from build123d import *

# Parameters (mm, degrees)
SKETCH1_W           = 42
SKETCH1_H           = 16
BOSS_EXTRUDE1_DEPTH = 7
SKETCH2_R           = 1
BOSS_EXTRUDE2_DEPTH = 1.6
CUT_EXTRUDE1_REACH  = 26.062
SKETCH3_R           = 1.45
BOSS_EXTRUDE3_DEPTH = 16
CUT_EXTRUDE2_REACH  = 72.718
SKETCH5_R           = 2.75
BOSS_EXTRUDE4_DEPTH = 6
CUT_EXTRUDE3_DEPTH  = 8
FILLET1_R           = 5
CHAMFER2_SIZE       = 3
CHAMFER3_SIZE       = 15
CHAMFER5_SIZE       = 20
SKETCH8_W           = 16
SKETCH8_H           = 4
SKETCH8_W_2         = 6
SKETCH8_H_2         = 10
CUT_EXTRUDE4_DEPTH  = 2
CHAMFER6_SIZE       = 2


with BuildPart() as part:
    # Sketch1 → Boss-Extrude1 (new body)
    with BuildSketch(Plane(origin=(0, 0, 0), x_dir=(1, 0, 0), z_dir=(0, 1, 0))):
        Rectangle(SKETCH1_W, SKETCH1_H)
    extrude(amount=BOSS_EXTRUDE1_DEPTH)

    # Sketch2 → Boss-Extrude2 (add)
    with BuildSketch(Plane(origin=(0, 7, 0), x_dir=(1, 0, 0), z_dir=(0, 1, 0))):
        with Locations(Location((-17, 5, 0), (0, 0, 270))):
            Circle(SKETCH2_R)
        with Locations(Location((-17, -5, 0), (0, 0, 270))):
            Circle(SKETCH2_R)
    extrude(amount=BOSS_EXTRUDE2_DEPTH)

    # Sketch3 → Cut-Extrude1 (cut, up to next)
    with BuildSketch(Plane(origin=(0, 0, 0), x_dir=(1, 0, 0), z_dir=(0, 1, 0)), mode=Mode.PRIVATE) as cut_extrude1_sk1:
        with Locations(Location((-2.5, 5, 0), (0, 0, 270))):
            Circle(SKETCH3_R)
    cut_extrude1_tool1 = extrude(cut_extrude1_sk1.sketch, amount=CUT_EXTRUDE1_REACH, mode=Mode.PRIVATE) & part.part
    # Sketch3 → Cut-Extrude1 (cut, up to next)
    with BuildSketch(Plane(origin=(0, 0, 0), x_dir=(1, 0, 0), z_dir=(0, 1, 0)), mode=Mode.PRIVATE) as cut_extrude1_sk2:
        with Locations(Location((17, 5, 0), (0, 0, 270))):
            Circle(SKETCH3_R)
    cut_extrude1_tool2 = extrude(cut_extrude1_sk2.sketch, amount=CUT_EXTRUDE1_REACH, mode=Mode.PRIVATE) & part.part
    add(cut_extrude1_tool1.solids().sort_by_distance((-2.5, 0, -5))[0], mode=Mode.SUBTRACT)
    add(cut_extrude1_tool2.solids().sort_by_distance((17, 0, -5))[0], mode=Mode.SUBTRACT)

    # Sketch4 → Boss-Extrude3 (add)
    with BuildSketch(Plane(origin=(0, 0, 0), x_dir=(1, 0, 0), z_dir=(0, 1, 0))):
        Polygon((-1, -8), (-21, -8), (-21, 8), (-61, 8), (-61, -32), (-1, -32), align=None)
    extrude(amount=BOSS_EXTRUDE3_DEPTH)

    # Sketch5 → Cut-Extrude2 (cut, up to next)
    with BuildSketch(Plane(origin=(0, 0, 0), x_dir=(1, 0, 0), z_dir=(0, 1, 0)), mode=Mode.PRIVATE) as cut_extrude2_sk1:
        with Locations(Location((-46, -17, 0), (0, 0, 270))):
            Circle(SKETCH5_R)
    cut_extrude2_tool1 = extrude(cut_extrude2_sk1.sketch, amount=CUT_EXTRUDE2_REACH, mode=Mode.PRIVATE) & part.part
    # Sketch5 → Cut-Extrude2 (cut, up to next)
    with BuildSketch(Plane(origin=(0, 0, 0), x_dir=(1, 0, 0), z_dir=(0, 1, 0)), mode=Mode.PRIVATE) as cut_extrude2_sk2:
        with Locations(Location((-16, -17, 0), (0, 0, 270))):
            Circle(SKETCH5_R)
    cut_extrude2_tool2 = extrude(cut_extrude2_sk2.sketch, amount=CUT_EXTRUDE2_REACH, mode=Mode.PRIVATE) & part.part
    add(cut_extrude2_tool1.solids().sort_by_distance((-46, 0, 17))[0], mode=Mode.SUBTRACT)
    add(cut_extrude2_tool2.solids().sort_by_distance((-16, 0, 17))[0], mode=Mode.SUBTRACT)

    # Sketch6 → Boss-Extrude4 (add)
    with BuildSketch(Plane(origin=(-40, 0, 0), x_dir=(0, 0, -1), z_dir=(1, 0, 0))):
        Polygon((-32, 0), (-42, 0), (-42, 16), (-35, 16), (-35, 13), (-37, 13), (-37, 5), (-32, 5), align=None)
    extrude(amount=-BOSS_EXTRUDE4_DEPTH)

    # Sketch7 → Cut-Extrude3 (cut)
    with BuildSketch(Plane(origin=(0, 16, 0), x_dir=(1, 0, 0), z_dir=(0, 1, 0))):
        Polygon((-21, 5), (-21, -5), (-29, -5), (-29, -32), (-35, -32), (-35, 5), align=None)
    extrude(amount=-CUT_EXTRUDE3_DEPTH, mode=Mode.SUBTRACT)

    # Fillet1
    fillet1_edges = [part.edges().sort_by_distance(p)[0] for p in [
        (-35, 12, -5),
        (-29, 12, 5),
        (-35, 12, 32),
    ]]
    fillet(fillet1_edges, radius=FILLET1_R)

    # Chamfer2
    chamfer2_edges = [part.edges().sort_by_distance(p)[0] for p in [
        (-34.5, 8, 32),
    ]]
    chamfer(chamfer2_edges, length=CHAMFER2_SIZE)

    # Chamfer3
    chamfer3_edges = [part.edges().sort_by_distance(p)[0] for p in [
        (-1, 8, 32),
        (-61, 8, 32),
    ]]
    chamfer(chamfer3_edges, length=CHAMFER3_SIZE)

    # Chamfer5
    chamfer5_edges = [part.edges().sort_by_distance(p)[0] for p in [
        (-61, 8, -8),
    ]]
    chamfer(chamfer5_edges, length=CHAMFER5_SIZE)

    # Sketch8 → Cut-Extrude4 (cut)
    with BuildSketch(Plane(origin=(0, 7, 0), x_dir=(1, 0, 0), z_dir=(0, 1, 0))):
        with Locations((7.5, -2)):
            Rectangle(SKETCH8_W, SKETCH8_H)
        with Locations((-8.5, 1)):
            Rectangle(SKETCH8_W_2, SKETCH8_H_2)
    extrude(amount=-CUT_EXTRUDE4_DEPTH, mode=Mode.SUBTRACT)

    # Chamfer6
    chamfer6_edges = [part.edges().sort_by_distance(p)[0] for p in [
        (7.5, 7, 4),
        (7.5, 7, 0),
        (-8.5, 7, 4),
        (-8.5, 5, -6),
    ]]
    chamfer(chamfer6_edges, length=CHAMFER6_SIZE - 0.0001)  # a hair under: the kernel refuses the full size


solid = part.part
Geometry: final body of the model. Coordinates: model frame, mm. A direction names the side the tool comes from. Coordinates: 2 decimals unless noted, no trailing zeros. Order: outer loops, then holes, each group sorted by start corner. A loop starts at its lowest first (then second) coordinate and runs counter-clockwise, first axis right, second up.
(1) Material intervals for probe 1 along X at (y, z) = (12, 17); probe 2 along X at (y, z) = (5.25, 17); probe 3 along Z at (x, y) = (-16, 9), sorted ascending.
(2) Section query A-A (x = 17). Return the cut outline in (y, z).
(3) First-contact query: pin 1 (5 mm diameter, centred on x = -10, z = -0.5, fed in from +Y); pin 2 (5 mm diameter, centred on x = -42.5, y = 8, fed in from -Z); pin 3 (5 mm diameter, centred on x = -16, z = 17, fed in from -Y); pin 4 (6.5 mm diameter, centred on x = -26, y = 13.5, fed in from +Z). Flat tips, straight axial feed; report the tip coordinate or a pass-through.
(4) Access query for faces 1 (the face through (-40, 6, 38)), 2 (the face through (-43, 15, 35)), 3 (the face through (-43, 13, 36)). Directions: +Z, -Z, +X, -X, +Y, -Y. A direction counts if a zero-diameter tool reaches every point of the face in a straight line with its end or side. Return the directions, or none.
(5) Draft query along X for faces 4 (the face through (-61, 8, 14)), 5 (the face through (-21, 0, 11)), 6 (the face through (-9, 5, 0)). Return one class per face: pulls with the +X half, pulls with the -X half, needs draft (parallel to the pull), parting line crosses it, or undercut.
(6) Section query B-B (z = 31). Return the cut outline in (x, y), plus the area to 3 significant figures.
(7) Section query D-D (y = 2.25). Return the cut outline in (x, z).
Solution:
1. probe 1: x = -61 to -48.75, -43.25 to -35, -29 to -18.75, -13.25 to -1
1. probe 2: x = -61 to -48.75, -43.25 to -18.75, -13.25 to -1
1. probe 3: z = 8 to 14.25, 19.75 to 32
2. outline: (0, -8) - (7, -8) - (7, -6.45) - (0, -6.45) - close; (0, -3.55) - (7, -3.55) - (7, 8) - (0, 8) - close
3. pin 1: stops at y = 7
3. pin 2: stops at z = -8
3. pin 3: passes through
3. pin 4: stops at z = 32
4. face 1: +Z, +X, +Y, -Y
4. face 2: +X, -X, +Y
4. face 3: +X, -X
5. face 4: pulls with the -X half
5. face 5: needs draft
5. face 6: undercut
6. outline: (-47, 0) - (-15, 0) - (-15, 16) - (-29, 16) - (-29, 6) - (-37, 6) - (-37, 16) - (-47, 16) - close
6. area: 432 mm2
7. outline: (-61, 12) - (-41, -8) - (21, -8) - (21, 8) - (-1, 8) - (-1, 17) - (-16, 32) - (-40, 32) - (-40, 42) - (-46, 42) - (-46, 32) - (-61, 17) - close; hole circle Ø5.5 at (-46, 17); hole circle Ø5.5 at (-16, 17); hole circle Ø2.9 at (-2.5, -5); hole circle Ø2.9 at (17, -5)
